from build123d import *

# Parameters (mm, degrees)
F1_DEPTH = 4
F2_DEPTH = 10
F3_DEPTH = 84
F4_R     = 0.5


with BuildPart() as f1:
    # F0 (on Top) → F1 (new body)
    with BuildSketch(Plane.XY):
        Polygon((71, -40), (71, 26.6875), (0, 40), (-71, 26.6875), (-71, -40), align=None)
        Polygon((77, -46), (77, 25.5625), (74, 26.125), (74, -43), (-74, -43), (-74, 26.125), (-77, 25.5625), (-77, -46), align=None)
        Polygon((0, 43), (71, 29.6875), (71, 32.6875), (0, 46), (-71, 32.6875), (-71, 29.6875), align=None)
        Polygon((-80, -49), (80, -49), (80, 25), (77, 25.5625), (77, -46), (-77, -46), (-77, 25.5625), (-80, 25), align=None)
        Polygon((74, -43), (74, 26.125), (71, 26.6875), (71, -40), (-71, -40), (-71, 26.6875), (-74, 26.125), (-74, -43), align=None)
        Polygon((-80, 31), (-80, 28), (-77, 28.5625), (-77, 31.5625), align=None)
        Polygon((-80, 34), (-80, 31), (-77, 31.5625), (-77, 34.5625), align=None)
        Polygon((-80, 28), (-80, 25), (-77, 25.5625), (-77, 28.5625), align=None)
        Polygon((-77, 34.5625), (-77, 31.5625), (-74, 32.125), (-74, 35.125), align=None)
        Polygon((-77, 31.5625), (-77, 28.5625), (-74, 29.125), (-74, 32.125), align=None)
        Polygon((-77, 28.5625), (-77, 25.5625), (-74, 26.125), (-74, 29.125), align=None)
        Polygon((-74, 32.125), (-74, 29.125), (-71, 29.6875), (-71, 32.6875), align=None)
        Polygon((-74, 29.125), (-74, 26.125), (-71, 26.6875), (-71, 29.6875), align=None)
        Polygon((-74, 35.125), (-74, 32.125), (-71, 32.6875), (-71, 35.6875), align=None)
        Polygon((0, 46), (71, 32.6875), (71, 35.6875), (0, 49), (-71, 35.6875), (-71, 32.6875), align=None)
        Polygon((0, 40), (71, 26.6875), (71, 29.6875), (0, 43), (-71, 29.6875), (-71, 26.6875), align=None)
        Polygon((71, 32.6875), (74, 32.125), (74, 35.125), (71, 35.6875), align=None)
        Polygon((74, 32.125), (77, 31.5625), (77, 34.5625), (74, 35.125), align=None)
        Polygon((77, 31.5625), (80, 31), (80, 34), (77, 34.5625), align=None)
        Polygon((77, 28.5625), (80, 28), (80, 31), (77, 31.5625), align=None)
        Polygon((77, 25.5625), (80, 25), (80, 28), (77, 28.5625), align=None)
        Polygon((74, 26.125), (77, 25.5625), (77, 28.5625), (74, 29.125), align=None)
        Polygon((71, 26.6875), (74, 26.125), (74, 29.125), (71, 29.6875), align=None)
        Polygon((71, 29.6875), (74, 29.125), (74, 32.125), (71, 32.6875), align=None)
        Polygon((74, 29.125), (77, 28.5625), (77, 31.5625), (74, 32.125), align=None)
    extrude(amount=F1_DEPTH)

    # F0 (on Top) → F2 (join)
    with BuildSketch(Plane.XY):
        Polygon((77, 31.5625), (80, 31), (80, 34), (77, 34.5625), align=None)
        Polygon((74, 32.125), (77, 31.5625), (77, 34.5625), (74, 35.125), align=None)
        Polygon((71, 32.6875), (74, 32.125), (74, 35.125), (71, 35.6875), align=None)
        Polygon((0, 46), (71, 32.6875), (71, 35.6875), (0, 49), (-71, 35.6875), (-71, 32.6875), align=None)
        Polygon((-74, 35.125), (-74, 32.125), (-71, 32.6875), (-71, 35.6875), align=None)
        Polygon((-77, 34.5625), (-77, 31.5625), (-74, 32.125), (-74, 35.125), align=None)
        Polygon((-80, 34), (-80, 31), (-77, 31.5625), (-77, 34.5625), align=None)
        Polygon((-80, 28), (-80, 25), (-77, 25.5625), (-77, 28.5625), align=None)
        Polygon((-77, 28.5625), (-77, 25.5625), (-74, 26.125), (-74, 29.125), align=None)
        Polygon((-74, 29.125), (-74, 26.125), (-71, 26.6875), (-71, 29.6875), align=None)
        Polygon((0, 40), (71, 26.6875), (71, 29.6875), (0, 43), (-71, 29.6875), (-71, 26.6875), align=None)
        Polygon((77, 25.5625), (80, 25), (80, 28), (77, 28.5625), align=None)
        Polygon((74, 26.125), (77, 25.5625), (77, 28.5625), (74, 29.125), align=None)
        Polygon((71, 26.6875), (74, 26.125), (74, 29.125), (71, 29.6875), align=None)
        Polygon((-80, -49), (80, -49), (80, 25), (77, 25.5625), (77, -46), (-77, -46), (-77, 25.5625), (-80, 25), align=None)
        Polygon((74, -43), (74, 26.125), (71, 26.6875), (71, -40), (-71, -40), (-71, 26.6875), (-74, 26.125), (-74, -43), align=None)
        Polygon((-80, 31), (-80, 28), (-77, 28.5625), (-77, 31.5625), align=None)
        Polygon((77, 28.5625), (80, 28), (80, 31), (77, 31.5625), align=None)
    extrude(amount=F2_DEPTH)

    # F0 (on Top) → F3 (join)
    with BuildSketch(Plane.XY):
        Polygon((77, -46), (77, 25.5625), (74, 26.125), (74, -43), (-74, -43), (-74, 26.125), (-77, 25.5625), (-77, -46), align=None)
        Polygon((-77, 28.5625), (-77, 25.5625), (-74, 26.125), (-74, 29.125), align=None)
        Polygon((74, 26.125), (77, 25.5625), (77, 28.5625), (74, 29.125), align=None)
    extrude(amount=F3_DEPTH)

    # F4
    f4_edges = [f1.edges().sort_by_distance(p)[0] for p in [
        (77, -8.71875, 84),
        (75.5, 28.84375, 84),
        (74, -6.9375, 84),
        (0, -43, 84),
        (-74, -6.9375, 84),
        (-75.5, 28.84375, 84),
        (-77, -8.71875, 84),
        (0, -46, 84),
    ]]
    fillet(f4_edges, radius=F4_R)


solid = f1.part
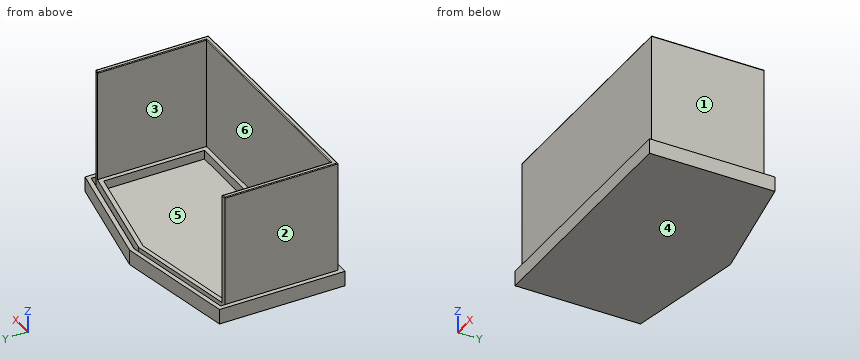
Verification items for the finished model (mm, model axes). Face numbers are marked on the shaded views. A direction names the side the tool comes from. Coordinates: 2 decimals unless noted, no trailing zeros. Order: outer loops, then holes, each group sorted by start corner. A loop starts at its lowest first (then second) coordinate and runs counter-clockwise, first axis right, second up. Notation, with made-up numbers: M 75.5,80 L 89.5,80 A3 cw 89.5,85 Z; hole C -25.75,64.25 d8. An arc over 180 degrees is marked long. Return JSON: item names as keys, results as strings.
1) Cross-section at D-D, the plane x = -54. Record the boundary of the cut face in (y, z) (3 decimals).
Answer list:
{"outline": "M -49,0 L 38.875,0 L 38.875,10 L 35.875,10 L 35.875,4 L 32.875,4 L 32.875,10 L 29.875,10 L 29.875,4 L -40,4 L -40,10 L -43,10 L -43,83.5 A0.5 ccw -43.5,84 L -45.5,84 A0.5 ccw -46,83.5 L -46,10 L -49,10 Z"}
2) Cross-section at C-C, the plane z = 55. Record the boundary of the cut face in (x, y) (1 decimal).
Answer list:
{"outline": "M -77,-46 L 77,-46 L 77,28.6 L 74,29.1 L 74,-43 L -74,-43 L -74,29.1 L -77,28.6 Z"}
3) Cross-section at A-A, the plane y = -6.5. Record the boundary of the cut face in (x, z), and give its area (3 significant figures).
Answer list:
{"outline": "M -80,0 L 80,0 L 80,10 L 77,10 L 77,83.5 A0.5 ccw 76.5,84 L 74.5,84 A0.5 ccw 74,83.5 L 74,10 L 71,10 L 71,4 L -71,4 L -71,10 L -74,10 L -74,83.5 A0.5 ccw -74.5,84 L -76.5,84 A0.5 ccw -77,83.5 L -77,10 L -80,10 Z", "area": "1,190 mm2"}
4) Cross-section at B-B, the plane x = -26. Record the boundary of the cut face in (y, z) (3 decimals), and give its area (3 significant figures).
Answer list:
{"outline": "M -49,0 L 44.125,0 L 44.125,10 L 41.125,10 L 41.125,4 L 38.125,4 L 38.125,10 L 35.125,10 L 35.125,4 L -40,4 L -40,10 L -43,10 L -43,83.5 A0.5 ccw -43.5,84 L -45.5,84 A0.5 ccw -46,83.5 L -46,10 L -49,10 Z", "area": "684 mm2"}
5) Thickness scan on L1, parallel to X at y = 12.5, z = 17.5; L2, parallel to X at y = 10.5, z = 8.5; L3, parallel to Z at x = 48.5, y = 29. Record the ranges inside material, lowest first. Write a range as [from, to].
Answer list:
{"L1": "[-77, -74], [74, 77]", "L2": "[-80, -71], [71, 80]", "L3": "[0, 4]"}
6) Access from +Z, -Z, +X, -X, +Y, -Y to the whole of each face (thin tool, end or side, straight path). Record for the marked faces 1, 2 and 3.
Answer list:
{"face 1": "+Z, +X, +Y, -Y", "face 2": "+Z, -X, +Y, -Y", "face 3": "+Z, +Y"}
7) Release check for a two-part mould opening along Y. For the marked faces 4, 5 and 6 record: +Y half, -Y half, draft (parallel to the pull), parting line (faces both ways), or undercut.
Answer list:
{"face 4": "draft", "face 5": "undercut", "face 6": "+Y half"}
8) Gauge pin test, flat ends, axial feed: pin 1 (12 mm diameter, centred on y = -36, z = 50, fed in from -X); pin 2 (6.5 mm diameter, centred on x = -17.5, z = 8, fed in from +Y); pin 3 (1 mm diameter, centred on x = -55, y = 25.5, fed in from +Z). Record the tip position at first contact, or that the pin passes through.
Answer list:
{"pin 1": "x = -77", "pin 2": "y = 46.33", "pin 3": "z = 4"}
